Input: part model. Units: mm. Frame: model coordinates. Face numbers are marked on the shaded views. Coordinates: 2 decimals unless noted, no trailing zeros. Order: outer loops, then holes, each group sorted by start corner. A loop starts at its lowest first (then second) coordinate and runs counter-clockwise, first axis right, second up. Notation, with made-up numbers: M 58.25,57.5 L 82.25,57.5 A30 ccw 82.25,91.5 Z; hole C 75,-31.75 d1. An arc over 180 degrees is marked long. One line per item, written item: value.
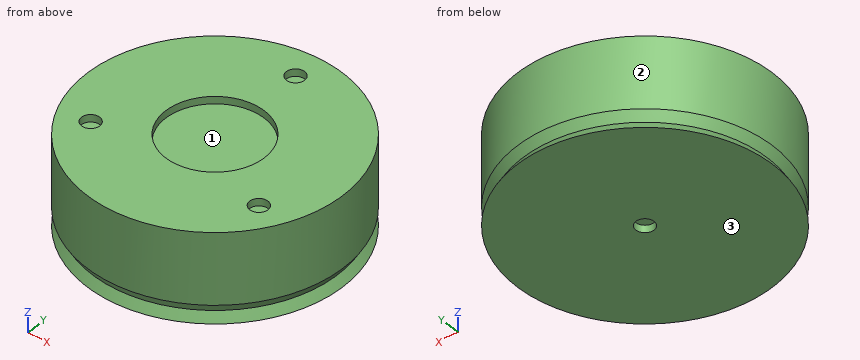
Autodesk Inventor part; units mm, degrees
ref_plane "작업 평면1" through (0, 0, -2.5) normal (0, 0, -1) x (-1, 0, 0)
ref_plane "작업 평면2" through (0, 0, -5) normal (0, 0, -1) x (-1, 0, 0)
ref_plane "YZ Plane" through (0, 0, 0) normal (1, 0, 0) x (0, 1, 0)
sketch "스케치1" plane through (0, 0, 0) normal (0, 0, 1) x (1, 0, 0)
  circle A0 centre (0, 0) radius 35
  dimension "d0" = 70
extrude "돌출1" add sketch "스케치1" along normal blind 19.5
sketch "스케치2" plane through (0, 0, 19.5) normal (0, 0, 1) x (1, 0, 0)
  line L0 (0, 0) -> (0, 27)
  circle A0 centre (0, 27) radius 2.5
  circle A1 centre (0, 0) radius 35
  circle A2 centre (-23.3827, -13.5) radius 2.5
  circle A3 centre (23.3827, -13.5) radius 2.5
  circle A4 centre (0, 0) radius 13.5
  dimension "d3" = 27
  dimension "d4" = 5
  dimension "d7" = 360
extrude "돌출2" cut sketch "스케치2" against normal blind 2 contours A0 | A2 | A3 | A4
ref_plane "작업 평면1" through (0, 0, -2.5) normal (0, 0, -1) x (-1, 0, 0)
sketch "스케치4" plane through (0, 0, -2.5) normal (0, 0, -1) x (-1, 0, 0)
  circle A0 centre (0, 0) radius 33.5
  dimension "d12" = 67
loft "로프트1" add profiles "스케치4" section 1 edges at (-35, 0, 0)
ref_plane "작업 평면2" through (0, 0, -5) normal (0, 0, -1) x (-1, 0, 0)
sketch "스케치5" plane through (0, 0, -5) normal (0, 0, -1) x (-1, 0, 0)
  circle A0 centre (0, 0) radius 35
  dimension "d18" = 70
loft "로프트2" add profiles "스케치5" section 1 edges at (-33.5, 0, -2.5)
sketch "스케치6" plane through (0, 0, -5) normal (0, 0, -1) x (-1, 0, 0)
  circle A0 centre (0, 0) radius 2.5
  dimension "d23" = 5
extrude "돌출3" cut sketch "스케치6" against normal blind 2
properties part number "sensor"
(1) Ray query, line 1 (Y direction, x = 0, z = 18.95); line 2 (X direction, y = 28.5, z = 18); line 3 (Z direction, x = -5, y = -2). Return the intervals inside material, ascending. Write a range as from..to.
Data:
line 1: y = -35..-13.5, 13.5..24.5, 29.5..35
line 2: x = -20.32..-2, 2..20.32
line 3: z = -5..17.5
(2) First-contact query: pin 1 (5 mm diameter, centred on x = -18, z = -1.5, fed in from -Y); pin 2 (8 mm diameter, centred on x = 4, y = -4, fed in from +Z); pin 3 (5 mm diameter, centred on y = 12.5, z = 16, fed in from +X). Flat tips, straight axial feed; report the tip coordinate or a pass-through.
Data:
pin 1: stops at y = -31.13
pin 2: stops at z = 17.5
pin 3: stops at x = 33.54
(3) Cut plane A-A on z = -1.5. Output: boundary loops of the cut face in (x, y), plus the area to 3 significant figures.
Data:
outline: C 0,0 d68.2
area: 3,650 mm2
(4) Draft query along Y for the marked faces 1, 2 and 3. Return one class per face: released by +Y, released by -Y, zero draft, split by the parting line, or undercut.
Data:
face 1: undercut
face 2: split by the parting line
face 3: zero draft
(5) Cut plane B-B on z = 13. Output: boundary loops of the cut face in (x, y), plus the area to 3 significant figures.
Data:
outline: C 0,0 d70
area: 3,850 mm2
